```python
from build123d import *

# Parameters (mm, degrees)
ESBO_O1_W                = 100
ESBO_O1_H                = 10
RESSALTO_EXTRUS_O1_DEPTH = 40
ESBO_O3_W                = 40
ESBO_O3_H                = 10
RESSALTO_EXTRUS_O2_DEPTH = 65
ESBO_O4_W                = 40
ESBO_O4_H                = 15
RESSALTO_EXTRUS_O3_DEPTH = 45
ESBO_O5_R                = 10
CORTE_EXTRUS_O1_DEPTH    = 90.582364336
ESBO_O7_R                = 15
CORTE_EXTRUS_O3_DEPTH    = 45
ESBO_O6_R                = 15
CORTE_EXTRUS_O4_DEPTH    = 21


with BuildPart() as part:
    # Esboço1 → Ressalto-extrusão1 (new body)
    with BuildSketch(Plane(origin=(0, 0, 0), x_dir=(1, 0, 0), z_dir=(0, 1, 0))):
        with Locations((0, 5)):
            Rectangle(ESBO_O1_W, ESBO_O1_H)
    extrude(amount=RESSALTO_EXTRUS_O1_DEPTH)

    # Esboço3 → Ressalto-extrusão2 (add)
    with BuildSketch(Plane(origin=(0, 0, -10), x_dir=(-1, 0, 0), z_dir=(0, 0, -1))):
        with Locations((0, 45)):
            Rectangle(ESBO_O3_W, ESBO_O3_H)
    extrude(amount=-RESSALTO_EXTRUS_O2_DEPTH)

    # Esboço4 → Ressalto-extrusão3 (add)
    with BuildSketch(Plane.XZ.offset(-40)):
        with Locations((0, 47.5)):
            Rectangle(ESBO_O4_W, ESBO_O4_H)
    extrude(amount=RESSALTO_EXTRUS_O3_DEPTH)

    # Esboço5 → Corte-extrusão1 (cut, through all)
    with BuildSketch(Plane.XY):
        with Locations((-30, 20)):
            Circle(ESBO_O5_R)
        with Locations((30, 20)):
            Circle(ESBO_O5_R)
        with Locations((0, 20)):
            Circle(ESBO_O5_R)
    extrude(amount=-CORTE_EXTRUS_O1_DEPTH, mode=Mode.SUBTRACT)

    # Esboço7 → Corte-extrusão3 (cut)
    with BuildSketch(Plane(origin=(0, 50, 0), x_dir=(1, 0, 0), z_dir=(0, 1, 0))):
        with Locations(Location((0, -20, 0), (0, 0, 270))):
            Circle(ESBO_O7_R)
    extrude(amount=-CORTE_EXTRUS_O3_DEPTH, mode=Mode.SUBTRACT)

    # Esboço6 → Corte-extrusão4 (cut)
    with BuildSketch(Plane.XY.offset(55)):
        with Locations((0, 20)):
            Circle(ESBO_O6_R)
    extrude(amount=-CORTE_EXTRUS_O4_DEPTH, mode=Mode.SUBTRACT)


solid = part.part
```
Model file for the job. Use its own axes, mm. A direction names the side the tool comes from. Coordinates: 2 decimals unless noted, no trailing zeros. Order: outer loops, then holes, each group sorted by start corner. A loop starts at its lowest first (then second) coordinate and runs counter-clockwise, first axis right, second up. Notation, with made-up numbers: (-33, 0) - (16, 0) arc R13 cw to (16, 5) - close; hole circle Ø3 at (-33, -14.75). An arc over 180 degrees is marked (long way). Return JSON: item names as keys, results as strings. Group by question number.
1) Saw through at B-B, the plane x = -30. Write the cut outline in (y, z), plus the area to 3 significant figures.
2) Saw through at A-A, the plane x = 0. Write the cut outline in (y, z), plus the area to 3 significant figures.
3) Flat gauge pins, fed straight in: P1, Ø24, axis at x = 0, z = 20, coming from the -Y side; P2, Ø3, axis at x = 24, z = -6.5, coming from the -Y side; P3, Ø3, axis at x = 36, y = 6, coming from the +Z side; P4, Ø2, axis at y = 2, z = 39.5, coming from the -X side. Where does each tip first touch, or does it go through?
4) Saw through at D-D, the plane z = 14.5. Write the cut outline in (x, y), plus the area to 3 significant figures.
5) Mould opens along Z. For faces 4 (the flat face through (-5, 35, 55)), 5 (the flat face through (-1, 0, -5)), 6 (the flat face through (-9, 40, 6)) say: released by +Z, released by -Z, zero draft, split by the parting line, or undercut.
6) Probe line 1 (Y direction, x = 30, z = -5.25); line 2 (Y direction, x = 0, z = 45.5); line 3 (Y direction, x = 16, z = 25.5). List the from-to ranges inside material, lowest first. Write a range as from..to.
7) Saw through at C-C, the plane y = 27. Write the cut outline in (x, z).
8) Tool access for faces 1 (the cylindrical face through (-3.252, 5.357, 47.605)), 2 (the flat face through (-35, 40, -5)), 3 (the flat face through (-9.2, 7.8, 40)): list every direction of +Z, -Z, +X, -X, +Y, -Y with a clear straight run to the whole face (end or side of a thin tool).
Values found:
{
 "1": {"outline": "(0, -10) - (10, -10) - (10, 0) - (0, 0) - close; (30, -10) - (40, -10) - (40, 0) - (30, 0) - close", "area": "200 mm²"},
 "2": {"outline": "(-5, 40) - (5, 40) - (5, 55) - (-5, 55) - close; (0, -10) - (10, -10) - (10, 0) - (0, 0) - close; (30, -10) - (50, -10) - (50, 5) - (40, 5) - (40, 0) - (30, 0) - close; (35, 40) - (40, 40) - (40, 35) - (50, 35) - (50, 55) - (35, 55) - close", "area": "775 mm²"},
 "3": {"P1": "passes through", "P2": "stops at y = 0", "P3": "stops at z = 0", "P4": "stops at x = -20"},
 "4": {"outline": "(-20, 40) - (-13.96, 40) - (-13.96, 50) - (-20, 50) - close; (13.96, 40) - (20, 40) - (20, 50) - (13.96, 50) - close", "area": "121 mm²"},
 "5": {"face 4": "released by +Z", "face 5": "zero draft", "face 6": "undercut"},
 "6": {"line 1": "y = 0..10, 30..40", "line 2": "y = -5..5, 35..50", "line 3": "y = 40..50"},
 "7": {"outline": "(-50, -10) - (-37.14, -10) - (-37.14, 0) - (-50, 0) - close; (-22.86, -10) - (-7.14, -10) - (-7.14, 0) - (-22.86, 0) - close; (-20, 40) - (-13.27, 40) - (-13.27, 55) - (-20, 55) - close; (7.14, -10) - (22.86, -10) - (22.86, 0) - (7.14, 0) - close; (13.27, 40) - (20, 40) - (20, 55) - (13.27, 55) - close; (37.14, -10) - (50, -10) - (50, 0) - (37.14, 0) - close"},
 "8": {"face 1": "+Z", "face 2": "+Z, -Z, -X, +Y", "face 3": "+X, -X, -Y"}
}
